CAD build for the part. Positions are in the model's coordinates, mm. Face numbers are marked on the shaded views. A direction names the side the tool comes from. Round coordinates to 2 decimals unless told otherwise and drop trailing zeros. Write each loop counter-clockwise with the first axis right and the second up, starting at its lowest first coordinate (ties: lowest second). Pieces come first, ordered by that corner, then holes. Notation, with made-up numbers: (-23.5, 18.5) - (0.5, 18.5) arc R30 ccw to (0.5, 43.5) - close; hole circle Ø11 at (52, 53). An arc over 180 degrees is marked (long way). Use one line per item in the form item = value. Start each with the question number.
Item 1: Tool access for the marked faces 4 and 5: list every direction of +Z, -Z, +X, -X, +Y, -Y with a clear straight run to the whole face (end or side of a thin tool).
Item 2: Pin check, flat tips, straight feed: pin 1 (1.5 mm diameter, centred on x = -9.5, z = -34, fed in from +Y); pin 2 (5.5 mm diameter, centred on x = -32, z = -11, fed in from +Y); pin 3 (5 mm diameter, centred on x = 30.5, y = 18, fed in from -Z). Stop position of each tip, or through.
Item 3: Drill centre lines: L1, parallel to X at y = 13, z = 0; L2, parallel to X at y = 4.85, z = 0; L3, parallel to X at y = 2.25, z = 21.5. Where is each one in solid material? Low to high.
Item 4: Band-saw the part on C-C, the plane x = -43.25. List the corners of the cut face in (y, z).
Item 5: Band-saw the part on B-B, the plane y = 10. List the corners of the cut face in (x, z), and give its area (3 significant figures).
Item 6: Band-saw the part on D-D, the plane z = 15.5. List the corners of the cut face in (x, y), and give its area (3 significant figures).
Item 7: Band-saw the part on A-A, the plane z = 0. List the corners of the cut face in (x, y).
Item 8: Pull direction X, two halves, no side cores. Call the marked faces 1, 2 and 3: +X half, -X half, draft (parallel to the pull), parting line (faces both ways), or undercut.
from build123d import *

# Parameters (mm, degrees)
SKETCH1_R                     = 47
BASE_BODY_DEPTH               = 21.5
SKETCH3_R                     = 39.5
CAVITY_DEPTH                  = 15.5
SKETCH4_R                     = 11.25
MOTOR_HOLE_DEPTH              = 69.251373613
MOTOR_SCREW_HOLES_D           = 3.6
MOTOR_SCREW_HOLES_CBORE_D     = 6.5
MOTOR_SCREW_HOLES_CBORE_DEPTH = 3.4
SKETCH8_R                     = 2.55
RING_PIN_HOLES_DEPTH          = 5
SKETCH9_R                     = 1.4
CAP_SCREW_HOLES_DEPTH         = 10


with BuildPart() as part:
    # Sketch1 → Base body (new body)
    with BuildSketch(Plane(origin=(0, 0, 0), x_dir=(1, 0, 0), z_dir=(0, 1, 0))):
        with Locations(Location((0, 0, 0), (0, 0, 270))):
            Circle(SKETCH1_R)
    extrude(amount=BASE_BODY_DEPTH)

    # Sketch3 → Cavity (cut)
    with BuildSketch(Plane(origin=(0, 21.5, 0), x_dir=(1, 0, 0), z_dir=(0, 1, 0))):
        with Locations(Location((0, 0, 0), (0, 0, 270))):
            Circle(SKETCH3_R)
    extrude(amount=-CAVITY_DEPTH, mode=Mode.SUBTRACT)

    # Sketch4 → Motor hole (cut, through all)
    with BuildSketch(Plane(origin=(0, 6, 0), x_dir=(1, 0, 0), z_dir=(0, 1, 0))):
        with Locations(Location((0, 0, 0), (0, 0, 270))):
            Circle(SKETCH4_R)
    extrude(amount=-MOTOR_HOLE_DEPTH, mode=Mode.SUBTRACT)

    # Motor screw holes (through all)
    with Locations(Plane(origin=(0, 6, 0), x_dir=(1, 0, 0), z_dir=(0, 1, 0))):
        with Locations((0, 0), (-15.5, -15.5), (15.5, 15.5), (15.5, -15.5), (-15.5, 15.5)):
            CounterBoreHole(MOTOR_SCREW_HOLES_D / 2, MOTOR_SCREW_HOLES_CBORE_D / 2, MOTOR_SCREW_HOLES_CBORE_DEPTH)

    # Sketch8 → Ring pin holes (cut)
    with BuildSketch(Plane(origin=(0, 6, 0), x_dir=(1, 0, 0), z_dir=(0, 1, 0))):
        with Locations(Location((-35, 0, 0), (0, 0, 270))):
            Circle(SKETCH8_R)
        with Locations(Location((-33.28697807, 10.815594803, 0), (0, 0, 270))):
            Circle(SKETCH8_R)
        with Locations(Location((-28.315594803, 20.57248383, 0), (0, 0, 270))):
            Circle(SKETCH8_R)
        with Locations(Location((-20.57248383, 28.315594803, 0), (0, 0, 270))):
            Circle(SKETCH8_R)
        with Locations(Location((-10.815594803, 33.28697807, 0), (0, 0, 270))):
            Circle(SKETCH8_R)
        with Locations(Location((0, 35, 0), (0, 0, 270))):
            Circle(SKETCH8_R)
        with Locations(Location((10.815594803, 33.28697807, 0), (0, 0, 270))):
            Circle(SKETCH8_R)
        with Locations(Location((20.57248383, 28.315594803, 0), (0, 0, 270))):
            Circle(SKETCH8_R)
        with Locations(Location((28.315594803, 20.57248383, 0), (0, 0, 270))):
            Circle(SKETCH8_R)
        with Locations(Location((33.28697807, 10.815594803, 0), (0, 0, 270))):
            Circle(SKETCH8_R)
        with Locations(Location((35, 0, 0), (0, 0, 270))):
            Circle(SKETCH8_R)
        with Locations(Location((33.28697807, -10.815594803, 0), (0, 0, 270))):
            Circle(SKETCH8_R)
        with Locations(Location((28.315594803, -20.57248383, 0), (0, 0, 270))):
            Circle(SKETCH8_R)
        with Locations(Location((20.57248383, -28.315594803, 0), (0, 0, 270))):
            Circle(SKETCH8_R)
        with Locations(Location((10.815594803, -33.28697807, 0), (0, 0, 270))):
            Circle(SKETCH8_R)
        with Locations(Location((0, -35, 0), (0, 0, 270))):
            Circle(SKETCH8_R)
        with Locations(Location((-10.815594803, -33.28697807, 0), (0, 0, 270))):
            Circle(SKETCH8_R)
        with Locations(Location((-20.57248383, -28.315594803, 0), (0, 0, 270))):
            Circle(SKETCH8_R)
        with Locations(Location((-28.315594803, -20.57248383, 0), (0, 0, 270))):
            Circle(SKETCH8_R)
        with Locations(Location((-33.28697807, -10.815594803, 0), (0, 0, 270))):
            Circle(SKETCH8_R)
    extrude(amount=-RING_PIN_HOLES_DEPTH, mode=Mode.SUBTRACT)

    # Sketch9 → Cap screw holes (cut)
    with BuildSketch(Plane(origin=(0, 21.5, 0), x_dir=(1, 0, 0), z_dir=(0, 1, 0))):
        with Locations(Location((-43.25, 0, 0), (0, 0, 270))):
            Circle(SKETCH9_R)
        with Locations(Location((-21.625, 37.455598714, 0), (0, 0, 270))):
            Circle(SKETCH9_R)
        with Locations(Location((21.625, 37.455598714, 0), (0, 0, 270))):
            Circle(SKETCH9_R)
        with Locations(Location((43.25, 0, 0), (0, 0, 270))):
            Circle(SKETCH9_R)
        with Locations(Location((21.625, -37.455598714, 0), (0, 0, 270))):
            Circle(SKETCH9_R)
        with Locations(Location((-21.625, -37.455598714, 0), (0, 0, 270))):
            Circle(SKETCH9_R)
    extrude(amount=-CAP_SCREW_HOLES_DEPTH, mode=Mode.SUBTRACT)


solid = part.part
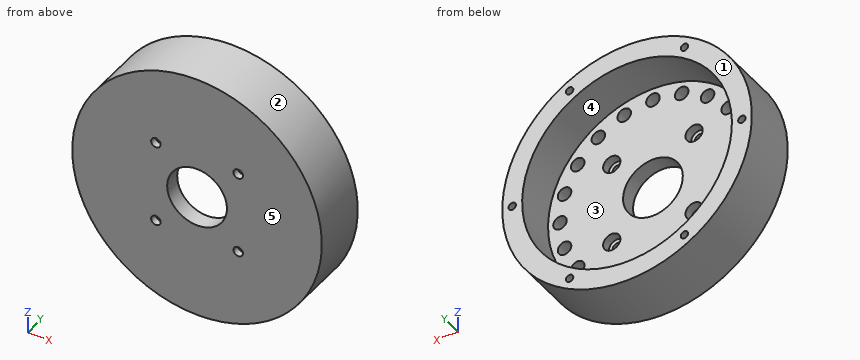
Determined:
q1.face_4 = +Y
q1.face_5 = +Z, -Z, +X, -X, -Y
q2.pin_1 = 1
q2.pin_2 = 6
q2.pin_3 = -37.75
q3.L1 = -47 to -44.65, -41.85 to -39.5, 39.5 to 41.85, 44.65 to 47
q3.L2 = -47 to -37.55, -32.45 to -11.25, 11.25 to 32.45, 37.55 to 47
q3.L3 = -41.79 to -30.69, -25.94 to 25.94, 30.69 to 41.79
q4.outline = (0, -18.4) - (21.5, -18.4) - (21.5, -1.4) - (11.5, -1.4) - (11.5, 1.4) - (21.5, 1.4) - (21.5, 18.4) - (0, 18.4) - close
q5.outline = circle Ø94 at (0, 0); hole circle Ø79 at (0, 0)
q5.area = 2,040 mm²
q6.outline = (-44.37, 0) - (-17.3, 0) - (-17.3, 2.6) - (-18.75, 2.6) - (-18.75, 6) - (-36.33, 6) - (-36.33, 21.5) - (-44.37, 21.5) - close; (-13.7, 0) - (13.7, 0) - (13.7, 2.6) - (12.25, 2.6) - (12.25, 6) - (-12.25, 6) - (-12.25, 2.6) - (-13.7, 2.6) - close; (17.3, 0) - (44.37, 0) - (44.37, 21.5) - (36.33, 21.5) - (36.33, 6) - (18.75, 6) - (18.75, 2.6) - (17.3, 2.6) - close
q6.area = 719 mm²
q7.outline = (-47, 0) - (-11.25, 0) - (-11.25, 6) - (-32.45, 6) - (-32.45, 1) - (-37.55, 1) - (-37.55, 6) - (-39.5, 6) - (-39.5, 21.5) - (-41.85, 21.5) - (-41.85, 11.5) - (-44.65, 11.5) - (-44.65, 21.5) - (-47, 21.5) - close; (11.25, 0) - (47, 0) - (47, 21.5) - (44.65, 21.5) - (44.65, 11.5) - (41.85, 11.5) - (41.85, 21.5) - (39.5, 21.5) - (39.5, 6) - (37.55, 6) - (37.55, 1) - (32.45, 1) - (32.45, 6) - (11.25, 6) - close
q8.face_1 = draft
q8.face_2 = parting line
q8.face_3 = undercut
